Autodesk Inventor part; units mm, degrees
ref_plane "YZ Plane" through (0, 0, 0) normal (1, 0, 0) x (0, 1, 0)
ref_plane "XZ Plane" through (0, 0, 0) normal (0, 1, 0) x (-1, 0, 0)
ref_plane "XY Plane" through (0, 0, 0) normal (0, 0, 1) x (1, 0, 0)
sketch "Sketch1" plane through (0, 0, 0) normal (0, 1, 0) x (-1, 0, 0)
  line L0 (0, 0) -> (0, 50.8)
  arc A0 (0, 50.8) -> (-58.7375, 109.5375) centre (-58.7375, 50.8) ccw
  line L1 (-58.7375, 109.5375) -> (-109.5375, 109.5375)
  line L2 (-58.7375, 109.5375) -> (0, 109.5375) construction
  line L3 (0, 109.5375) -> (0, 50.8) construction
  dimension "d0" = 109.5375
  dimension "d1" = 109.5375
  dimension "d2" = 50.8
sketch "Sketch2" plane through (0, 0, 0) normal (0, 0, 1) x (1, 0, 0)
  circle A0 centre (0, 0) radius 57.8231
  circle A1 centre (0, 0) radius 50.3047
  dimension "d3" = 100.6094
  dimension "d4" = 115.6462
sweep "Sweep1" add profiles "Sketch2" path "Sketch1"
sketch "Sketch3" plane through (0, 0, 0) normal (0, 0, -1) x (-1, 0, 0)
  circle A0 centre (0, 0) radius 63.3984
  circle A1 centre (0, 0) radius 57.8231
  circle A2 centre (0, 0) radius 54.0639
  dimension "d6" = 126.7968
  dimension "d9" = 108.1278
extrude "Extrusion1" add sketch "Sketch3" against normal blind 56.8198 contours A0 | A1
sketch "Sketch4" plane through (109.5375, 0, 109.5375) normal (1, 0, 0) x (0, 0, -1)
  circle A0 centre (0, 0) radius 50.3047
  circle A1 centre (0, 0) radius 54.0639
  circle A2 centre (0, 0) radius 63.3984
  dimension "d10" = 126.7968
  dimension "d11" = 108.1278
extrude "Extrusion2" add sketch "Sketch4" against normal blind 56.8198 contours A2
sketch "Sketch5" plane through (0, 0, 0) normal (0, 0, -1) x (-1, 0, 0)
  circle A0 centre (0, 0) radius 50.3047
  circle A1 centre (0, 0) radius 57.3786
  dimension "d14" = 114.7572
sketch "Sketch5 outline for Extrusion3" plane through (0, 0, 0) normal (0, 0, -1) x (-1, 0, 0)
  circle A0 centre (0, 0) radius 57.3786
extrude "Extrusion3" cut sketch "Sketch5 outline for Extrusion3" against normal blind 50.8 draft -0.38674
sketch "Sketch6" plane through (109.5375, 0, 109.5375) normal (1, 0, 0) x (0, 0, -1)
  circle A0 centre (0, 0) radius 50.3047
  circle A1 centre (0, 0) radius 57.3786
  dimension "d17" = 114.7572
sketch "Sketch6 outline for Extrusion4" plane through (109.5375, 0, 109.5375) normal (1, 0, 0) x (0, 0, -1)
  circle A0 centre (0, 0) radius 57.3786
extrude "Extrusion4" cut sketch "Sketch6 outline for Extrusion4" against normal blind 50.8 draft -0.38674
equation "\"d0\" = G + C1"
equation "\"d1\" = G + C1"
equation "\"d2\" = C1"
equation "\"d3\" = D"
equation "\"d4\" = D + 2 * F1"
equation "\"d6\" = A + 2 * E1"
equation "\"d9\" = D + F1"
equation "\"d7\" = C1 + E1"
equation "\"d10\" = A + 2 * E1"
equation "\"d11\" = D + F1"
equation "\"d12\" = C1 + E1"
equation "\"d14\" = A"
equation "\"d15\" = C1"
equation "\"d17\" = A"
equation "\"d18\" = C1"
equation "\"A\" = 114.7572"
equation "\"C1\" = 50.8"
equation "\"F1\" = 7.5184"
equation "\"D\" = 100.6094"
equation "\"G\" = 58.7375"
equation "\"E1\" = 6.0198"
equation "\"B\" = 114.0714"
properties part number "ASTM D 2466 90 Deg Elbow Socket-Type - Schedule 40 4" material "PVC-Piping"
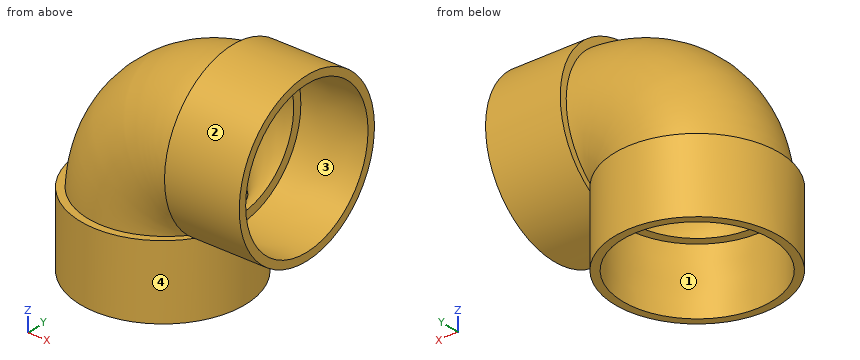
Check sheet for the modelled part. Datum: model origin and axes. Units: mm. Face numbers are marked on the shaded views. A direction names the side the tool comes from. Give positions to 0.01 mm unless a question says otherwise; leave off trailing zeros. Order: outer loops, then holes, each group sorted by start corner. A loop starts at its lowest first (then second) coordinate and runs counter-clockwise, first axis right, second up. Notation, with made-up numbers: M 21,28.5 L 68,28.5 A20 ccw 68,62.5 Z; hole C 32.25,-28 d9. An arc over 180 degrees is marked long. Answer in a Markdown table with one row per item. Add a question column.
Q1. Gauge pin test, flat ends, axial feed: pin 1 Ø6 at (x, y) = (90, 8.5) entering from -Z; pin 2 Ø10 at (x, z) = (31, 95.5) entering from +Y; pin 3 Ø2 at (y, z) = (15.5, 47) entering from -X. Record the tip position at first contact, or that the pin passes through.
Q2. Sectioned sample at A-A, the plane x = 61. Record the boundary of the cut face in (y, z), and give its area (3 significant figures).
Q3. Thickness scan on L1, parallel to Y at x = 56.5, z = 98; L2, parallel to Y at x = 102, z = 135.5; L3, parallel to Z at x = 78, y = -12.5. Record the ranges inside material, lowest first.
Q4. Sectioned sample at C-C, the plane x = 83. Record the boundary of the cut face in (y, z), and give its area (3 significant figures).
Q5. Access from +Z, -Z, +X, -X, +Y, -Y to the whole of each face (thin tool, end or side, straight path). Record for the marked faces 1 and 2.
Q6. Release check for a two-part mould opening along Y. For the marked faces 3 and 4 record: released by +Y, released by -Y, zero draft, split by the parting line, or undercut.
Q7. Sectioned sample at B-B, the plane y = 31.5. Count the separate pieces of the cut face and the enclosed holes in it, and give its area (3 significant figures).
Verdict:
| question | item | result |
|---|---|---|
| 1 | pin 1 | z = 46.38 |
| 1 | pin 2 | y = 57.81 |
| 1 | pin 3 | x = -61.72 |
| 2 | outline | M -17.27,0 L 17.27,0 L 17.27,48.54 A63.4 ccw long -17.27,48.54 Z; hole C 0,109.54 d114.1 |
| 2 | area | 4,020 mm² |
| 3 | L1 | -62.34 to -48.98, 48.98 to 62.34 |
| 3 | L2 | -57.84 to -51.11, 51.11 to 57.84 |
| 3 | L3 | 47.38 to 53.76, 165.32 to 171.69 |
| 4 | outline | C 0,109.54 d126.8; hole C 0,109.54 d114.4 |
| 4 | area | 2,350 mm² |
| 5 | face 1 | -Z |
| 5 | face 2 | +X |
| 6 | face 3 | undercut |
| 6 | face 4 | split by the parting line |
| 7 | separate pieces | 2 |
| 7 | enclosed holes | 1 |
| 7 | area | 3,330 mm² |
